The figure shows three views and two pictorial views of one solid part (mm, origin at its lowest corner). Answer the questions. Round coordinates to 2 decimals unless told otherwise and drop trailing zeros. Write each loop counter-clockwise with the first axis right and the second up, starting at its lowest first coordinate (ties: lowest second). Pieces come first, ordered by that corner, then holes.
Item 1: Find section D-D on y = 120. Give the vertices of the cut face in (x, z), then the cut area to 3 significant figures.
Item 2: Find the intervals of material crossed by probe 1 along Y at (x, z) = (225.5, 15); probe 2 along X at (y, z) = (504, 16.5); probe 3 along X at (y, z) = (92, 80.5), in increasing order.
Item 3: Find section A-A on x = 204. Give the vertices of the cut face in (y, z), then the cut area to 3 significant figures.
Item 4: Find section C-C on z = 7.5. Give the number of separate pieces and of enclosed holes in the cut face, then the cut area to 3 significant figures.
Item 5: Find section B-B on y = 258. Give the vertices of the cut face in (x, z).
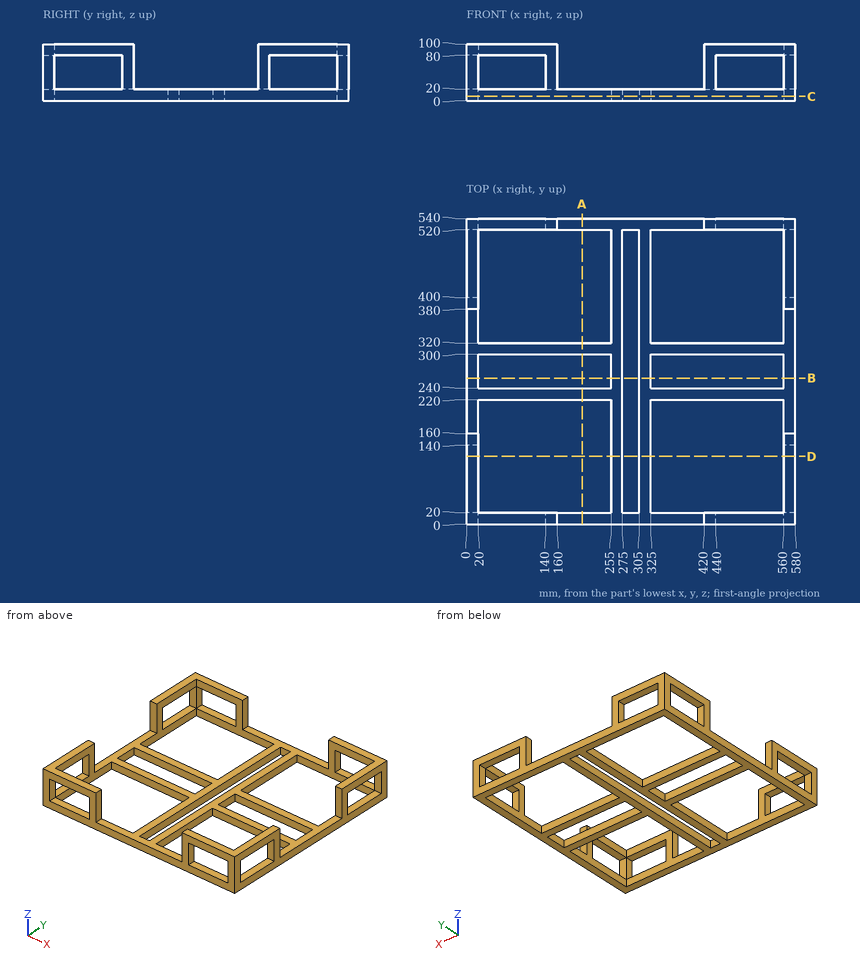
Check values:
1. outline: (0, 0) - (20, 0) - (20, 20) - (0, 20) - close; (0, 80) - (20, 80) - (20, 100) - (0, 100) - close; (255, 0) - (275, 0) - (275, 20) - (255, 20) - close; (305, 0) - (325, 0) - (325, 20) - (305, 20) - close; (560, 0) - (580, 0) - (580, 20) - (560, 20) - close; (560, 80) - (580, 80) - (580, 100) - (560, 100) - close
1. area: 2,400 mm2
2. probe 1: y = 0 to 20, 220 to 240, 300 to 320, 520 to 540
2. probe 2: x = 0 to 20, 255 to 275, 305 to 325, 560 to 580
2. probe 3: x = 0 to 20, 560 to 580
3. outline: (0, 0) - (20, 0) - (20, 20) - (0, 20) - close; (220, 0) - (240, 0) - (240, 20) - (220, 20) - close; (300, 0) - (320, 0) - (320, 20) - (300, 20) - close; (520, 0) - (540, 0) - (540, 20) - (520, 20) - close
3. area: 1,600 mm2
4. separate pieces: 1
4. enclosed holes: 7
4. area: 82,000 mm2
5. outline: (0, 0) - (20, 0) - (20, 20) - (0, 20) - close; (255, 0) - (275, 0) - (275, 20) - (255, 20) - close; (305, 0) - (325, 0) - (325, 20) - (305, 20) - close; (560, 0) - (580, 0) - (580, 20) - (560, 20) - close
